The drawing under review shows one solid part. Ordinate dimensions are in mm from its lowest x, y, z. Round coordinates to 2 decimals unless told otherwise and drop trailing zeros. Loops run counter-clockwise (first coordinate to the right, second up) from the corner with the lowest first, then second, coordinate; pieces in that order, holes last. Notation, with made-up numbers: M -19.5,-22.75 L -6.5,-22.75 A25 cw -6.5,-10.75 Z; hole C -14,58 d9. An arc over 180 degrees is marked long. Use a Markdown table: item, result.
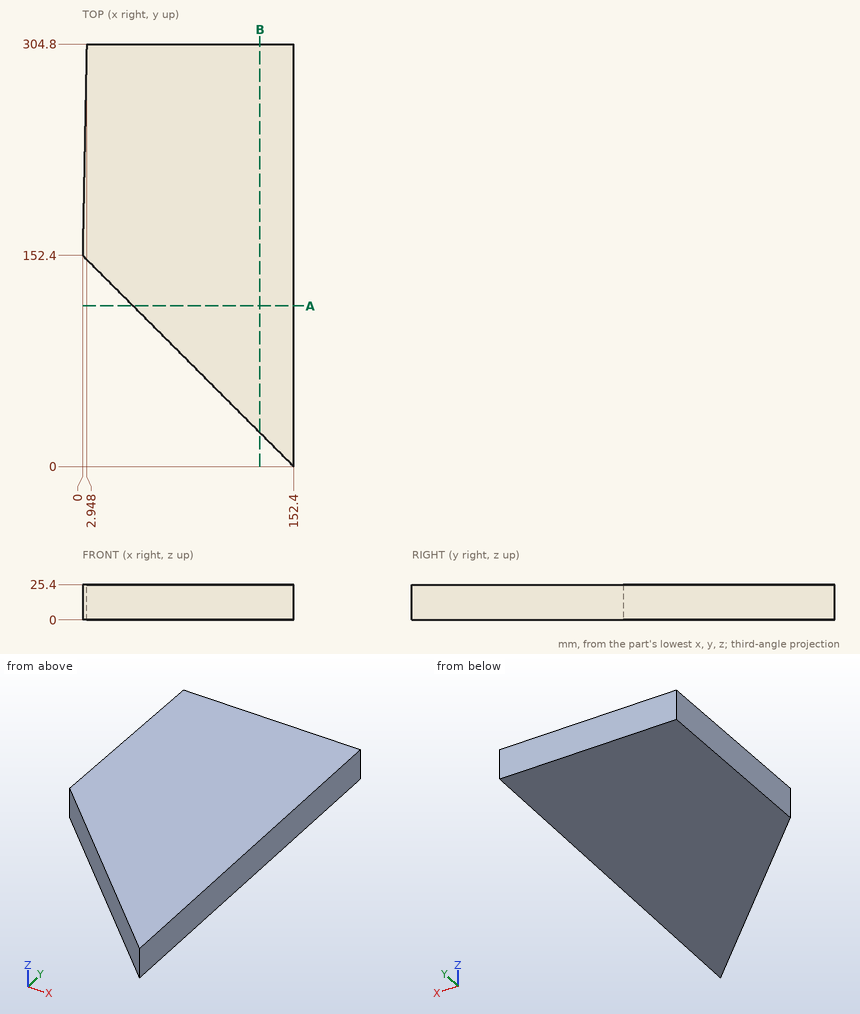
1. Insertion check: pin 1 (4 mm diameter, centred on x = 129, z = 8, fed in from -Y); pin 2 (1 mm diameter, centred on y = 200.5, z = 6.5, fed in from -X); pin 3 (10 mm diameter, centred on y = 213, z = 17.5, fed in from -X). Each pin has a flat end and moves straight along its axis. Give the tip position at first contact, or say it passes through.
Check values:
| item | result |
|---|---|
| pin 1 | stops at y = 21.4 |
| pin 2 | stops at x = 0.92 |
| pin 3 | stops at x = 1.08 |
2. Take a section at B-B on x = 128. Give the boundary of the cut face in (y, z).
Check values:
| item | result |
|---|---|
| outline | M 24.4,0 L 304.8,0 L 304.8,25.4 L 24.4,25.4 Z |
3. Wall thickness on line 1 along X through (y, z) = (246.5, 11.5); line 2 along Y through (x, z) = (66, 8.25); line 3 along Y through (x, z) = (123, 17.75): over which ranges is each line inside the solid? List them lowest first. Write a range as from..to.
Check values:
| item | result |
|---|---|
| line 1 | x = 1.82..152.4 |
| line 2 | y = 86.4..304.8 |
| line 3 | y = 29.4..304.8 |
4. Take a section at A-A on y = 116. Give the boundary of the cut face in (x, z).
Check values:
| item | result |
|---|---|
| outline | M 36.4,0 L 152.4,0 L 152.4,25.4 L 36.4,25.4 Z |
